```python
from build123d import *

# Parameters (mm, degrees)
SCHIZZO1_W                   = 10
SCHIZZO1_H                   = 4
ESTRUSIONE_ESTRUSIONE3_DEPTH = 4


with BuildPart() as part:
    # Schizzo1 → Estrusione-Estrusione3 (new body)
    with BuildSketch(Plane.XY):
        with BuildLine():
            Line((400, 30), (400, 0))
            Line((400, 0), (700, 0))
            Line((700, 0), (700, 30))
            Line((700, 30), (700, 73))
            ThreePointArc((700, 73), (697.949747468, 77.949747468), (693, 80))
            Line((693, 80), (654.193736081, 80))
            ThreePointArc((654.193736081, 80), (652.382002765, 79.761480784), (650.693736081, 79.062177826))
            Line((650.693736081, 79.062177826), (581.959107885, 39.378221735))
            ThreePointArc((581.959107885, 39.378221735), (565.076441043, 32.38519216), (546.959107885, 30))
            Line((546.959107885, 30), (400, 30))
        make_face()
        with Locations((450, 23)):
            Rectangle(SCHIZZO1_W, SCHIZZO1_H, mode=Mode.SUBTRACT)
        with Locations((550, 23)):
            Rectangle(SCHIZZO1_W, SCHIZZO1_H, mode=Mode.SUBTRACT)
        with Locations((650, 23)):
            Rectangle(SCHIZZO1_W, SCHIZZO1_H, mode=Mode.SUBTRACT)
        with BuildLine():
            Line((690, 63), (690, 37))
            ThreePointArc((690, 37), (687.949747468, 32.050252532), (683, 30))
            Line((683, 30), (611.839907009, 30))
            ThreePointArc((611.839907009, 30), (605.078426225, 35.188266684), (608.339907009, 43.062177826))
            Line((608.339907009, 43.062177826), (653.373228005, 69.062177826))
            ThreePointArc((653.373228005, 69.062177826), (655.06149469, 69.761480784), (656.873228005, 70))
            Line((656.873228005, 70), (683, 70))
            ThreePointArc((683, 70), (687.949747468, 67.949747468), (690, 63))
        make_face(mode=Mode.SUBTRACT)
    extrude(amount=ESTRUSIONE_ESTRUSIONE3_DEPTH)


solid = part.part
```
The listing builds one solid part. Answer for the finished solid, in the listing's coordinates (mm). A direction names the side the tool comes from. Coordinates: 2 decimals unless noted, no trailing zeros. Write each loop counter-clockwise with the first axis right and the second up, starting at its lowest first coordinate (ties: lowest second). Pieces come first, ordered by that corner, then holes. Notation, with made-up numbers: (33, 59) - (60, 59) arc R18 ccw to (60, 68) - close; hole circle Ø9 at (7, 29). An arc over 180 degrees is marked (long way). Return JSON: item names as keys, results as strings. Group by question number.
1. A cutting plane is placed at A-A, the plane z = 2.35. Give the number of separate pieces and of enclosed holes in the cut face, plus the area to 3 significant figures.
2. Given pin 1 (1.2 mm diameter, centred on x = 448.5, z = 1.5, fed in from -Y); pin 2 (1.5 mm diameter, centred on x = 624, z = 3, fed in from +Y); pin 3 (1.2 mm diameter, centred on x = 449.5, z = 3, fed in from +Y); pin 4 (1.2 mm diameter, centred on x = 649, z = 1, fed in from +Y), each flat-ended and moving along its own axis, determine where each tip first touches the part or whether it passes through.
3. A cutting plane is placed at D-D, the plane x = 558.5. Determine the outline of the cut face in (y, z), plus the area to 3 significant figures.
4. Determine the mould class of faces 1 (the cylindrical face through (698, 77.9, 2)), 2 (the cylindrical face through (687.9, 68, 2)), 3 (the flat face through (572, 25, 0)), 4 (the flat face through (630.54, 55.88, 1.97)) for opening direction X: released by +X, released by -X, zero draft, split by the parting line, or undercut.
5. Which of the six approach directions +Z, -Z, +X, -X, +Y, -Y give full straight-line access (tool end or side, diameter ignored) to faces 5 (the cylindrical face through (605.113, 35.065, 1.972)), 6 (the flat face through (572, 25, 4))?
6. A cutting plane is placed at B-B, the plane x = 674. Determine the outline of the cut face in (y, z).
7. A cutting plane is placed at C-C, the plane x = 448.5. Determine the outline of the cut face in (y, z), plus the area to 3 significant figures.
8. Straight lines are drawn through the part: L1, parallel to X at y = 23, z = 3.25; L2, parallel to Y at x = 681, z = 2.4; L3, parallel to X at y = 59.5, z = 1.9. For each, find the intervals that lie inside material, in ascending order.
Ans:
{
 "1": {"separate pieces": "1", "enclosed holes": "4", "area": "10,800 mm²"},
 "2": {"pin 1": "y = 0", "pin 2": "y = 64.08", "pin 3": "y = 30", "pin 4": "y = 78.43"},
 "3": {"outline": "(0, 0) - (30.96, 0) - (30.96, 4) - (0, 4) - close", "area": "124 mm²"},
 "4": {"face 1": "released by +X", "face 2": "undercut", "face 3": "zero draft", "face 4": "undercut"},
 "5": {"face 5": "+Z, -Z", "face 6": "+Z, +X, -X, +Y, -Y"},
 "6": {"outline": "(0, 0) - (30, 0) - (30, 4) - (0, 4) - close; (70, 0) - (80, 0) - (80, 4) - (70, 4) - close"},
 "7": {"outline": "(0, 0) - (21, 0) - (21, 4) - (0, 4) - close; (25, 0) - (30, 0) - (30, 4) - (25, 4) - close", "area": "104 mm²"},
 "8": {"L1": "400 to 445, 455 to 545, 555 to 645, 655 to 700", "L2": "0 to 30, 70 to 80", "L3": "616.81 to 636.81, 690 to 700"}
}
